Input: part model. Units: mm. Frame: model coordinates. A direction names the side the tool comes from. Give positions to 0.01 mm unless a question says otherwise; leave off trailing zeros. Order: outer loops, then holes, each group sorted by start corner. A loop starts at its lowest first (then second) coordinate and runs counter-clockwise, first axis right, second up. Notation, with made-up numbers: (45.25, -29) - (75.25, -29) arc R34 ccw to (75.25, 4) - close; hole circle Ø6 at (73, 48). An arc over 180 degrees is marked (long way). Answer in a Markdown table with one row per item. Add a question column.
1. Access query for faces 1 (the face through (-7, 7, 25.4)), 2 (the face through (23, 25.4, 3)), 3 (the face through (12, 10, 0)), 4 (the face through (4, 25.4, 22)), 5 (the face through (32, 7, 25.4)). Directions: +Z, -Z, +X, -X, +Y, -Y. A direction counts if a zero-diameter tool reaches every point of the face in a straight line with its end or side. Return the directions, or none.
2. Section query B-B on x = 12.7. Return loops of the section in (y, z), and give its area (3 significant figures).
3. Contact query for flat-ended pins moving along their axis: pin 1 (12.5 mm diameter, centred on x = 33.5, y = 18.5, fed in from +Z); pin 2 (6 mm diameter, centred on y = 7.5, z = 40.5, fed in from -X); pin 3 (5 mm diameter, centred on y = 33, z = 12.5, fed in from +X). Output: stop coordinate, or through.
4. Ray query, line 1 (Z direction, x = -18, y = 3.5); line 2 (Z direction, x = 14, y = 7). Return the intervals inside material, ascending. Write a range as [from, to].
5. Section query D-D on z = 23. Return loops of the section in (x, y), and give its area (3 significant figures).
6. Section query A-A on y = 23. Return loops of the section in (x, z).
7. Section query C-C on z = 11. Return loops of the section in (x, y).
Autodesk Inventor part; units mm, degrees
ref_plane "Work Plane1" through (0, 0, 25.4) normal (0, 0, 1) x (1, 0, 0)
ref_plane "YZ Plane" through (0, 0, 0) normal (1, 0, 0) x (0, 1, 0)
ref_plane "XZ Plane" through (0, 0, 0) normal (0, 1, 0) x (-1, 0, 0)
sketch "Sketch1" plane through (0, 0, 0) normal (0, 0, 1) x (1, 0, 0)
  line L0 (0, 0) -> (25.4, 0)
  line L1 (25.4, 0) -> (25.4, 25.4)
  line L2 (25.4, 25.4) -> (0, 25.4)
  line L3 (0, 25.4) -> (0, 0)
  line L4 (25.4, 0) -> (50.8, 0)
  line L5 (50.8, 0) -> (25.4, 25.4)
  line L6 (0, 0) -> (-25.4, 0)
  line L7 (-25.4, 0) -> (0, 25.4)
  dimension "d0" = 25.4
  dimension "d1" = 25.4
  dimension "d2" = 25.4
  dimension "d3" = 25.4
extrude "Extrusion1" add sketch "Sketch1" along normal blind 25.4 contours L3 L2 L1 L0
chamfer "Chamfer1" distance 0.3 angle 45 2 edges at (25.4, 12.7, 25.4) (0, 12.7, 25.4)
sketch "Sketch2" plane through (0, 0, 25.4) normal (0, 0, 1) x (1, 0, 0)
  line L0 (0, 0) -> (-25.4, 0)
  line L1 (0, 25.4) -> (0, 0)
  line L2 (-25.4, 0) -> (0, 25.4)
  line L3 (25.4, 0) -> (50.8, 0)
  line L4 (50.8, 0) -> (25.4, 25.4)
  dimension "d9" = 25.4
  dimension "d10" = 25.4
extrude "Extrusion2" add sketch "Sketch2" against normal blind 25.4
sketch "Sketch3" plane through (0, 0, 25.4) normal (0, 0, 1) x (1, 0, 0)
  line L0 (-25.4, 0) -> (25.4, 0)
  line L1 (25.4, 0) -> (50.8, 0)
  line L2 (25.4, 0) -> (25.4, 25.4)
  line L3 (50.8, 0) -> (25.4, 25.4)
  point P0 (0, 0)
  dimension "d13" = 25.4
extrude "Extrusion3" add sketch "Sketch3" against normal blind 25.4
sketch "Sketch4" plane through (0, 0, 25.4) normal (0, 0, 1) x (1, 0, 0)
  line L0 (0.3, 0) -> (25.1, 0)
  circle A0 centre (12.7, 0) radius 12.7
  point P0 (0, 0)
  dimension "d16" = 25.4
extrude "Extrusion4" add sketch "Sketch4" along normal blind 25.4
ref_plane "Work Plane1" through (0, 0, 25.4) normal (0, 0, 1) x (1, 0, 0)
sketch "Sketch5" plane through (0, 0, 25.4) normal (0, 0, 1) x (1, 0, 0)
  line L0 (0, 0) -> (-25.4, 0)
  line L1 (0, 0) -> (42.4435, 0)
  line L2 (42.4435, 0) -> (42.4435, -16.3705)
  line L3 (42.4435, -16.3705) -> (0, -16.3705)
  line L4 (0, -16.3705) -> (0, 0)
  circle A0 centre (12.7, 0) radius 12.7
extrude "Extrusion5" cut sketch "Sketch5" along normal blind 25.4 contours A0 L1 L2 L3 L4 | L1 A0 picked at (10.2952, -3.484)
sketch "Sketch6" plane through (0.3, 25.4, 25.4) normal (0, 1, 0) x (1, 0, 0)
  point P0 (-0.3, 25.4)
sketch "Sketch7" plane through (0.3, 25.4, 25.4) normal (0, 1, 0) x (1, 0, 0)
  point P0 (-0.3, 25.4)
sketch "Sketch8" plane through (0.3, 25.4, 25.4) normal (0, 1, 0) x (1, 0, 0)
  circle A0 centre (12.7153, 12.8448) radius 12.7
  point P0 (-0.3, 25.4)
  dimension "d22" = 25.4
extrude "Extrusion6" add sketch "Sketch8" along normal blind 25.4
properties part number "orthographic1"
Answer:
| question | item | result |
|---|---|---|
| 1 | face 1 | +Z, -X, +Y, -Y |
| 1 | face 2 | -Z, +X, +Y |
| 1 | face 3 | -Z, +X, -X, -Y |
| 1 | face 4 | +Y |
| 1 | face 5 | +Z, +X, +Y, -Y |
| 2 | outline | (0, 0) - (25.4, 0) - (25.4, -0.14) - (50.8, -0.14) - (50.8, 25.25) - (25.4, 25.25) - (25.4, 25.4) - (12.7, 25.4) - (12.7, 50.8) - (0, 50.8) - close |
| 2 | area | 1,610 mm² |
| 3 | pin 1 | stops at z = 25.4 |
| 3 | pin 2 | stops at x = 0.82 |
| 3 | pin 3 | stops at x = 25.72 |
| 4 | line 1 | z = [0, 25.4] |
| 4 | line 2 | z = [0, 50.8] |
| 5 | outline | (-25.4, 0) - (50.8, 0) - (25.4, 25.4) - (20.24, 25.4) - (20.24, 50.8) - (5.79, 50.8) - (5.79, 25.4) - (0, 25.4) - close |
| 5 | area | 1,660 mm² |
| 6 | outline | (-2.4, 0) - (27.8, 0) - (27.8, 25.4) - (25.4, 25.4) - (25.4, 25.1) - (25.1, 25.4) - (0.3, 25.4) - (0, 25.1) - (0, 25.4) - (-2.4, 25.4) - close |
| 7 | outline | (-25.4, 0) - (50.8, 0) - (25.4, 25.4) - (25.62, 25.4) - (25.62, 50.8) - (0.41, 50.8) - (0.41, 25.4) - (0, 25.4) - close |
